```python
from build123d import *

# Parameters (mm, degrees)
F0_W      = 30
F0_H      = 19
F1_DEPTH  = 10.5
F3_DEPTH  = 4.35
F6_DEPTH  = 12.5
F7_DEPTH  = 10.5
F9_DEPTH  = 5.25
F11_DEPTH = 10.5


with BuildPart() as f1:
    # F0 (on Front) → F1 (new body, symmetric)
    with BuildSketch(Plane.XZ):
        with Locations((-40.8455379754, 6.5018872991)):
            Rectangle(F0_W, F0_H)
    extrude(amount=F1_DEPTH, both=True)

    # F2 (on Front) → F3 (cut, symmetric)
    with BuildSketch(Plane.XZ):
        Polygon((-39.8867149711, 0), (-31.6867149711, 0), (-31.6867149711, 10.7), (-39.8867149711, 11.8163746178), (-39.8550798476, 12.8947440535), (-48.5550798476, 12.8947440535), (-48.5708974093, 14.4973720267), (-48.5867149711, 16.1), (-56.2867149711, 16.1), (-56.2867149711, 0), align=None)
        Polygon((-31.6346511245, -4.0566790849), (-31.6867149711, 0), (-39.8867149711, 0), (-56.2867149711, 0), (-56.2867149711, -4.0566790849), align=None)
        Polygon((-48.5550798476, 12.8947440535), (-39.8550798476, 12.8947440535), (-48.5708974093, 14.4973720267), align=None)
    extrude(amount=F3_DEPTH, both=True, mode=Mode.SUBTRACT)

    # F5 (on Top) → F6 (cut, symmetric)
    with BuildSketch(Plane.XY):
        Polygon((-31.664647162, -3.3765389722), (-45.2137924731, -4.4331237346), (-31.664647162, -4.4641996406), align=None)
        Polygon((-31.664647162, 4.4641996406), (-45.2137924731, 4.4331237346), (-31.664647162, 3.3765389722), align=None)
    extrude(amount=F6_DEPTH, both=True, mode=Mode.SUBTRACT)

    # F4 (on Front) → F7 (cut, symmetric)
    with BuildSketch(Plane.XZ):
        with BuildLine():
            Line((-45.7834748578, 16.0856869832), (-56.2834748578, 16.0856869832))
            Line((-56.2834748578, 16.0856869832), (-56.2834748578, 5.1856869832))
            Line((-56.2834748578, 5.1856869832), (-45.7834748578, 5.1856869832))
            ThreePointArc((-45.7834748578, 5.1856869832), (-41.9297429004, 6.7819550257), (-40.3334748578, 10.6356869832))
            ThreePointArc((-40.3334748578, 10.6356869832), (-41.9297429004, 14.4894189406), (-45.7834748578, 16.0856869832))
        make_face()
        with BuildLine():
            Line((-40.3334748578, 16.0856869832), (-45.7834748578, 16.0856869832))
            ThreePointArc((-45.7834748578, 16.0856869832), (-41.9297429004, 14.4894189406), (-40.3334748578, 10.6356869832))
            Line((-40.3334748578, 10.6356869832), (-40.3334748578, 16.0856869832))
        make_face()
    extrude(amount=F7_DEPTH, both=True, mode=Mode.SUBTRACT)

    # F8 (on Front) → F9 (join, symmetric)
    with BuildSketch(Plane.XZ):
        Polygon((-36.0005199909, 18.7051203102), (-56.4405918121, 18.7051203102), (-56.4405918121, 16.7337413877), (-47.9325428605, 16.7337413877), (-47.9325428605, 15.0736346841), (-41.1883555353, 13.7247974053), (-36.0005199909, 13.7247974053), align=None)
    extrude(amount=F9_DEPTH, both=True)

    # F10 (on Front) → F11 (join, symmetric)
    with BuildSketch(Plane.XZ):
        Polygon((-13.3185807616, 16.0780958831), (-25.8185807616, 16.0780958831), (-30.0829801708, 16.0780958831), (-22.8185807616, -91.9219041169), (-13.3185807616, -91.9219041169), align=None)
    extrude(amount=F11_DEPTH, both=True)


solid = f1.part
```
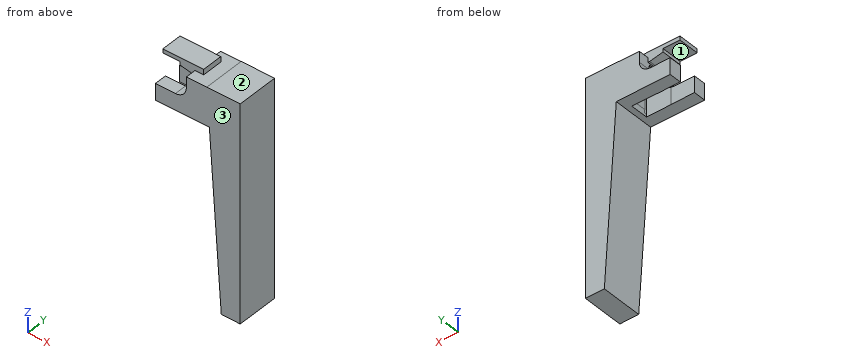
Here's how the part is built. I have some questions about the finished solid (model axes, mm). Face numbers are marked on the shaded views. A direction names the side the tool comes from. Coordinates: 2 decimals unless noted, no trailing zeros. Loops run counter-clockwise (first coordinate to the right, second up) from the corner with the lowest first, then second, coordinate; pieces in that order, holes last. Notation, with made-up numbers: (75.5, 73.25) - (85.5, 73.25) arc R24 cw to (85.5, 89.25) - close; hole circle Ø5 at (71.5, 87.5). An arc over 180 degrees is marked (long way). Return JSON: item names as keys, results as strings. Group by question number.
Item 1: I need wall thicknesses on line 1 (Z direction, x = -53.5, y = 4.5); line 2 (Z direction, x = -21, y = 6.5); line 3 (Z direction, x = -29.5, y = -2). Which ranges of each line are inside material? Lowest first, please. Write a range as from..to.
Item 2: Will these pins go through, and if not, where does the flat tip stop? P1, Ø0.9, axis at x = -41, y = -1, coming from the -Z side; P2, Ø2, axis at x = -31.5, y = 7, coming from the -Z side; P3, Ø7, axis at y = 7.5, z = 1.5, coming from the -X side; P4, Ø5, axis at x = -50.5, y = 7.5, coming from the +Z side.
Item 3: If we section it at D-D on x = -33.5: Write out the boundary of the cut face in (y, z), and give its area (3 significant figures).
Item 4: On a 3-axis mill with a long thin cutter (end or side, diameter ignored), from which of +Z, -Z, +X, -X, +Y, -Y can I reach the whole of each face in a straight line? I mean the marked faces 1, 2 and 3. Say none if no direction works.
Item 5: If we section it at A-A on x = -49.5: Write out the boundary of the cut face in (y, z).
Item 6: If we section it at C-C on y = -7.5: Write out the boundary of the cut face in (x, z).
Calculated:
{
 "1": {"line 1": "z = -3..5.19, 16.73..18.71", "line 2": "z = -91.92..16.08", "line 3": "z = -3..16.08"},
 "2": {"P1": "stops at z = 13.72", "P2": "stops at z = -3", "P3": "stops at x = -55.85", "P4": "stops at z = 18.71"},
 "3": {"outline": "(-10.5, -3) - (-4.46, -3) - (-4.46, 12.5) - (-3.52, 12.5) - (-3.52, 10.95) - (3.52, 10.95) - (3.52, 12.5) - (4.46, 12.5) - (4.46, -3) - (10.5, -3) - (10.5, 16) - (-10.5, 16) - close", "area": "272 mm^2"},
 "4": {"face 1": "-X, +Y, -Y", "face 2": "+Z, +X, +Y, -Y", "face 3": "+Z, -Z, +X, -X, -Y"},
 "5": {"outline": "(-10.5, -3) - (-4.35, -3) - (-4.35, 5.19) - (-10.5, 5.19) - close; (-5.25, 16.73) - (5.25, 16.73) - (5.25, 18.71) - (-5.25, 18.71) - close; (4.35, -3) - (10.5, -3) - (10.5, 5.19) - (4.35, 5.19) - close"},
 "6": {"outline": "(-55.85, -3) - (-28.8, -3) - (-22.82, -91.92) - (-13.32, -91.92) - (-13.32, 16.08) - (-30.08, 16.08) - (-30.08, 16) - (-40.33, 16) - (-40.33, 10.64) arc R5.45 cw to (-45.78, 5.19) - (-55.85, 5.19) - close"}
}
